Autodesk Inventor part; units mm, degrees
ref_plane "YZ Plane" through (0, 0, 0) normal (1, 0, 0) x (0, 1, 0)
ref_plane "XZ Plane" through (0, 0, 0) normal (0, 1, 0) x (-1, 0, 0)
ref_plane "XY Plane" through (0, 0, 0) normal (0, 0, 1) x (1, 0, 0)
sketch "Boceto1" plane through (0, 0, 0) normal (0, 0, 1) x (1, 0, 0)
  line L0 (-28, 0) -> (28, 0)
  line L1 (-28, 0) -> (-28, 13)
  line L2 (-28, 13) -> (-20.6795, 25.6795)
  line L3 (-20.6795, 25.6795) -> (15.3205, 25.6795)
  line L4 (15.3205, 25.6795) -> (28, 13)
  line L5 (28, 13) -> (28, 0)
  line L6 (15.3205, 25.6795) -> (15.3205, 18.6795)
  line L7 (-24.7209, 18.6795) -> (22.3205, 18.6795) construction
  point P0 (0, 0)
  dimension "d0" = 28
  dimension "d1" = 28
  dimension "d2" = 13
  dimension "d3" = 36
  dimension "d4" = 135
  dimension "d6" = 7
  dimension "d16" = 150
extrude "Extrusión1" add sketch "Boceto1" along normal mid plane 18
sketch "Boceto2" plane through (-20.6795, 25.6795, 9) normal (0, 1, 0) x (1, 0, 0)
  line L0 (-7.3205, 18) -> (-7.3205, 0) construction
  line L1 (-7.3205, 12) -> (48.6795, 12) construction
  line L2 (48.6795, 18) -> (48.6795, 0) construction
  line L3 (-7.3205, 6) -> (48.6795, 6) construction
  line L4 (0, 18) -> (36, 18) construction
  line L5 (-4.0415, 12) -> (-4.0415, 6)
  line L6 (43, 12) -> (43, 6)
  line L7 (-4.0415, 12) -> (43, 12)
  line L8 (43, 6) -> (-4.0415, 6)
  point P0 (20.6795, 9)
  point P1 (-4.0415, 9)
  point P2 (43, 9)
  dimension "d9" = 6
  dimension "d10" = 6
extrude "Extrusión2" cut sketch "Boceto2" against normal blind 7
The model under review builds one solid part; all positions refer to its coordinate system, in mm. A direction names the side the tool comes from. Give positions to 0.01 mm unless a question says otherwise; leave off trailing zeros. Order: outer loops, then holes, each group sorted by start corner. A loop starts at its lowest first (then second) coordinate and runs counter-clockwise, first axis right, second up. Notation, with made-up numbers: (-25, 38) -> (-2, 38) arc R29 cw to (-2, 69) -> close; hole circle Ø10 at (36.5, 49). An arc over 180 degrees is marked (long way). Write item = value, one per line. Start each with the question number.
(1) For L1, parallel to Z at x = 7.5, y = 19.25; L2, parallel to Y at x = -16.5, z = -1; L3, parallel to Y at x = 25.5, z = -1.25, list the stretches that pass through material, from the lowest coordinate up. Write a range as from..to.
(2) Take a section at B-B (y = 20). Write out the cut boundary in (x, z), plus the area to 3 significant figures.
(3) For pin 1 Ø5 at (x, z) = (8.5, 0) entering from +Y; pin 2 Ø2 at (y, z) = (15.5, 5.5) entering from -X, all flat-tipped, find the tip position at first contact; note any pin that passes through.
(4) Take a section at D-D (x = -10). Write out the cut boundary in (y, z).
(5) Take a section at C-C (z = -4.75). Write out the cut boundary in (x, y), plus the area to 3 significant figures.
(6) Tool access review of faces 4 (the flat face through (-2, 22, -3)), 5 (the flat face through (-3, 25.68, 6)): name each direction out of +Z, -Z, +X, -X, +Y, -Y from which nothing blocks a thin tool from reaching the whole face with its end or side.
(7) Take a section at A-A (x = 19.5). Write out the cut boundary in (y, z), plus the area to 3 significant figures.
(8) Draft analysis for pull direction Z (two halves, no side actions). For faces 1 (the flat face through (0, 0, 0)), 2 (the flat face through (-2, 18.68, 0)), 3 (the flat face through (0, 13, -9)), state which applies: +Z half, -Z half, draft (parallel to the pull), parting line (faces both ways), or undercut.
Returned:
q1.L1 = -9..-3, 3..9
q1.L2 = 0..18.68
q1.L3 = 0..15.5
q2.outline = (-23.96, -9) -> (21, -9) -> (21, -3) -> (-23.96, -3) -> close; (-23.96, 3) -> (21, 3) -> (21, 9) -> (-23.96, 9) -> close
q2.area = 540 mm²
q3.pin_1 = 18.68
q3.pin_2 = -27.13
q4.outline = (0, -9) -> (25.68, -9) -> (25.68, -3) -> (18.68, -3) -> (18.68, 3) -> (25.68, 3) -> (25.68, 9) -> (0, 9) -> close
q5.outline = (-28, 0) -> (28, 0) -> (28, 13) -> (15.32, 25.68) -> (-20.68, 25.68) -> (-28, 13) -> close
q5.area = 1,310 mm²
q6.face_4 = +X, -X, +Y
q6.face_5 = +Z, -Z, +X, -X, +Y
q7.outline = (0, -9) -> (21.5, -9) -> (21.5, -3) -> (18.68, -3) -> (18.68, 3) -> (21.5, 3) -> (21.5, 9) -> (0, 9) -> close
q7.area = 370 mm²
q8.face_1 = draft
q8.face_2 = undercut
q8.face_3 = -Z half
